Geometry: see drawing. Coordinates: mm, zero at the bounding-box minimum. A direction names the side the tool comes from. Give positions to 0.01 mm unless a question says otherwise; leave off trailing zeros. Write each loop counter-clockwise with the first axis right and the second up, starting at its lowest first coordinate (ties: lowest second). Pieces come first, ordered by that corner, then holes. Notation, with made-up numbers: (18, 39) -> (45, 39) arc R20 cw to (45, 49) -> close; hole circle Ø8 at (24.25, 22). An arc over 180 degrees is marked (long way). Answer as a JSON object with one key per item and string values. Group by question number.
Item 1: Section query C-C on z = 12.5. Return the cut outline in (x, y), plus the area to 3 significant figures.
Item 2: Ray query, probe 1 along X at (y, z) = (9, 19); probe 2 along Y at (x, z) = (295, 9.5); probe 3 along Z at (x, y) = (186, 49). Return the intervals inside material, ascending. Write a range as from..to.
Item 3: First-contact query: pin 1 Ø21.5 at (x, y) = (59, 15.5) entering from -Z; pin 2 Ø3 at (x, z) = (433.5, 49) entering from +Y; pin 3 Ø20 at (y, z) = (13.5, 14.5) entering from -X. Flat tips, straight axial feed; report the tip coordinate or a pass-through.
Item 4: Section query D-D on y = 53.5. Return the cut outline in (x, z).
Item 5: Access query for the marked faces 1, 2 and 3. Directions: +Z, -Z, +X, -X, +Y, -Y. A direction counts if a zero-diameter tool reaches every point of the face in a straight line with its end or side. Return the directions, or none.
Item 6: Section query B-B on y = 14. Return the cut outline in (x, z).
Item 7: Section query A-A on x = 157. Return the cut outline in (y, z).
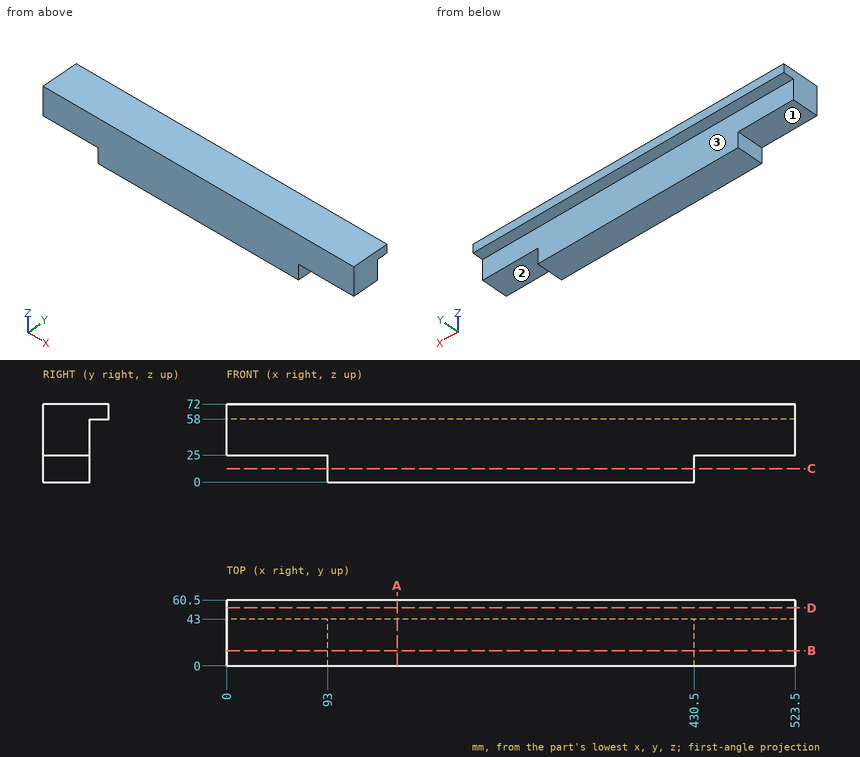
Worked answers:
{
 "1": {"outline": "(93, 0) -> (430.5, 0) -> (430.5, 43) -> (93, 43) -> close", "area": "14,500 mm^2"},
 "2": {"probe 1": "93..430.5", "probe 2": "0..43", "probe 3": "58..72"},
 "3": {"pin 1": "z = 25", "pin 2": "y = 43", "pin 3": "x = 93"},
 "4": {"outline": "(0, 58) -> (523.5, 58) -> (523.5, 72) -> (0, 72) -> close"},
 "5": {"face 1": "-Z, -X, +Y, -Y", "face 2": "-Z, +X, +Y, -Y", "face 3": "-Z, +X, -X, +Y"},
 "6": {"outline": "(0, 25) -> (93, 25) -> (93, 0) -> (430.5, 0) -> (430.5, 25) -> (523.5, 25) -> (523.5, 72) -> (0, 72) -> close"},
 "7": {"outline": "(0, 0) -> (43, 0) -> (43, 58) -> (60.5, 58) -> (60.5, 72) -> (0, 72) -> close"}
}
